from build123d import *

# Parameters (mm, degrees)
SKETCH1_W               = 25.4
SKETCH1_H               = 2.7432
BOSS_EXTRUDE1_DEPTH     = 203.2
CUT_EXTRUDE1_DEPTH      = 109.054860552
CUT_EXTRUDE1_DEPTH_BACK = 109.054860552
SKETCH2_R               = 3.96875


with BuildPart() as part:
    # Sketch1 → Boss-Extrude1 (new body)
    with BuildSketch(Plane(origin=(0, 0, 0), x_dir=(1, 0, 0), z_dir=(0, 1, 0))):
        with Locations((12.7, -1.3716)):
            Rectangle(SKETCH1_W, SKETCH1_H)
    extrude(amount=BOSS_EXTRUDE1_DEPTH)

    # Sketch2 → Cut-Extrude1 (cut, two sides: drawn at the far end of the back side and taken through both)
    with BuildSketch(Plane(origin=(8.791703067, 106.606717755, 5.9182), x_dir=(1, 0, 0), z_dir=(0, 0, 1)).offset(-CUT_EXTRUDE1_DEPTH_BACK)):
        with Locations((3.908296933, 64.843282245)):
            Circle(SKETCH2_R)
        with Locations(Location((3.908296933, -74.856717755, 0), (0, 0, 180))):
            Circle(SKETCH2_R)
    extrude(amount=CUT_EXTRUDE1_DEPTH + CUT_EXTRUDE1_DEPTH_BACK, mode=Mode.SUBTRACT)


solid = part.part
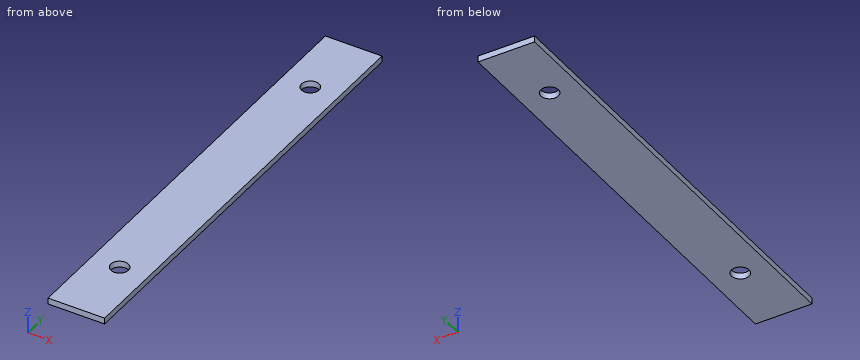
Read the model definition and answer for the solid it produces. Units are mm, in the model's axes. Round coordinates to 2 decimals unless told otherwise and drop trailing zeros. Write each loop counter-clockwise with the first axis right and the second up, starting at its lowest first coordinate (ties: lowest second). Pieces come first, ordered by that corner, then holes. Notation, with made-up numbers: (19, -1.75) - (71, -1.75) arc R31 cw to (71, 25.25) - close; hole circle Ø11 at (16, 70). An arc over 180 degrees is marked (long way). Use a Markdown table: item, result.
(1) This flat-tipped pin is pushed along its axis until it touches: pin 1 Ø9 at (x, y) = (12.7, 171.45) entering from -Z. Where does it stop, or does it pass through?
Reported:
| item | result |
|---|---|
| pin 1 | z = 0 |
(2) The part is cut by section C-C (z = 0.5). Write down the section's boundary in (x, y).
Reported:
| item | result |
|---|---|
| outline | (0, 0) - (25.4, 0) - (25.4, 203.2) - (0, 203.2) - close; hole circle Ø7.94 at (12.7, 31.75); hole circle Ø7.94 at (12.7, 171.45) |
(3) The part is cut by section B-B (y = 31.75). Write down the section's boundary in (x, z).
Reported:
| item | result |
|---|---|
| outline | (0, 0) - (8.73, 0) - (8.73, 2.74) - (0, 2.74) - close; (16.67, 0) - (25.4, 0) - (25.4, 2.74) - (16.67, 2.74) - close |
(4) The part is cut by section A-A (x = 12.7). Write down the section's boundary in (y, z), then the cut area to 3 significant figures.
Reported:
| item | result |
|---|---|
| outline | (0, 0) - (27.78, 0) - (27.78, 2.74) - (0, 2.74) - close; (35.72, 0) - (167.48, 0) - (167.48, 2.74) - (35.72, 2.74) - close; (175.42, 0) - (203.2, 0) - (203.2, 2.74) - (175.42, 2.74) - close |
| area | 514 mm2 |
(5) Straight lines are drawn through the part: line 1 along Y through (x, z) = (12.7, 1.8); line 2 along X through (y, z) = (171.45, 1.3); line 3 along Y through (x, z) = (13.75, 2). For each, find the intervals that lie inside material, in ascending order. Write a range as [from, to].
Reported:
| item | result |
|---|---|
| line 1 | [0, 27.78], [35.72, 167.48], [175.42, 203.2] |
| line 2 | [0, 8.73], [16.67, 25.4] |
| line 3 | [0, 27.92], [35.58, 167.62], [175.28, 203.2] |
